```python
from build123d import *

# Parameters (mm, degrees)
PAD008_DEPTH      = 9.5
POCKET004_DEPTH   = 7
POCKET005_DEPTH   = 7.3
PAD009_DEPTH      = 4.1
PAD009_DEPTH_BACK = 9.5
PAD010_DEPTH      = 9.5
SKETCH019_R       = 2.1
PAD011_DEPTH      = 3


with BuildPart() as part:
    # Sketch012 → Pad008 (new body, symmetric)
    with BuildSketch(Plane.YZ):
        Polygon((-50.2140974459, 25.1635701276), (-41.6041734691, 21.1486966411), (-32.9942494922, 17.1338231546), (-30.6406576873, 16.391738509), (-21.2849840337, 14.7420808212), (-11.9293103801, 13.0924231333), (-9.4638496319, 12.9847787924), (0, 13.8127583485), (9.4638496319, 14.6407379046), (11.8731622478, 15.1748696522), (20.8002421453, 18.4240610138), (29.7273220427, 21.6732523754), (31.9162958532, 22.8127600157), (39.698240274, 28.261736161), (47.4801846947, 33.7107123064), (49.7744904401, 30.4341041292), (34.2106015986, 19.5361518385), (31.0954026161, 17.9144818923), (13.2412428211, 11.4160991691), (9.8124726029, 10.6559591122), (-9.1152266609, 9), (-12.6239030908, 9.1531921213), (-31.335250398, 12.4525074969), (-34.6847225392, 13.5085920064), (-51.9045704929, 21.5383389795), align=None)
    extrude(amount=PAD008_DEPTH, both=True)

    # Sketch013 → Pocket004 (cut, symmetric)
    with BuildSketch(Plane.YZ):
        Polygon((45.432304584, 32.2767712155), (39.698240274, 28.261736161), (33.9641759639, 24.2467011065), (34.7671886347, 23.0998922076), (33.7022888371, 22.3542413419), (35.1935840518, 20.2244435621), (41.9925460194, 24.9851279839), (48.791507987, 29.7458124056), (47.3002178304, 31.8756137271), (46.2353203941, 31.1299645148), align=None)
        Polygon((27.3780904908, 20.8182020171), (20.8002421453, 18.4240610138), (14.2223937998, 16.0299200105), (14.701229209, 14.7143529651), (13.4796275966, 14.2697263401), (14.3688739661, 11.826523341), (22.1683227186, 14.6652905307), (29.9677714711, 17.5040577203), (29.078530336, 19.9472626244), (27.8569308195, 19.5026367622), align=None)
        Polygon((-6.9733628866, 13.2026681492), (-6.8513426496, 11.8079957641), (-8.1463884643, 11.6946939366), (-7.9197930232, 9.1045868913), (0.348622971, 9.8279795561), (8.6170389652, 10.5513722209), (8.390436117, 13.1414786182), (7.0953826538, 13.0281761215), (6.9733628866, 14.4228485477), (0, 13.8127583485), align=None)
        Polygon((-21.2849840337, 14.7420808212), (-28.1786383048, 15.9576180648), (-28.4217503954, 14.5788880291), (-29.701997863, 14.8046301996), (-30.1534810944, 12.2441296837), (-21.9795767444, 10.8028498091), (-13.8056723944, 9.3615699345), (-13.3541906242, 11.922070708), (-14.6344528215, 12.1478154758), (-14.3913297626, 13.5265435775), align=None)
        Polygon((-41.6041734691, 21.1486966411), (-47.9483279783, 24.1070244733), (-48.5400033464, 22.838198142), (-49.7182011739, 23.3876008118), (-50.8170011484, 21.0311970654), (-43.294646516, 17.523465493), (-35.7722918836, 14.0157339205), (-34.6734914189, 16.3721374383), (-35.8516963311, 16.9215434118), (-35.2600189598, 18.1903688089), align=None)
    extrude(amount=POCKET004_DEPTH, both=True, mode=Mode.SUBTRACT)

    # Sketch014 → Pocket005 (cut, symmetric)
    with BuildSketch(Plane.YZ):
        Polygon((27.8569308195, 19.5026367622), (27.7885250582, 19.6905746558), (14.6328241506, 14.9022911145), (14.701229209, 14.7143529651), (13.4796275966, 14.2697263401), (13.7532418641, 13.5179715711), (29.3521429929, 19.1955072693), (29.078530336, 19.9472626244), align=None)
        Polygon((7.0779512585, 13.2274150395), (7.0953826538, 13.0281761215), (8.390436117, 13.1414786182), (8.4601600703, 12.3445228037), (-8.0766667901, 10.8977379227), (-8.1463884643, 11.6946939366), (-6.8513426496, 11.8079957641), (-6.8687741121, 12.0072346763), align=None)
        Polygon((34.6524725388, 23.2637220503), (46.1206038498, 31.2937940434), (46.2353203941, 31.1299645148), (47.3002178304, 31.8756137271), (47.7590763401, 31.2202902435), (34.1611489031, 21.6989189481), (33.7022888371, 22.3542413419), (34.7671886347, 23.0998922076), align=None)
        Polygon((-48.5400033464, 22.838198142), (-49.7182011739, 23.3876008118), (-50.0562934738, 22.6625535052), (-35.0115838696, 15.6470902021), (-34.6734914189, 16.3721374383), (-35.8516963311, 16.9215434118), (-35.7671709924, 17.1028041826), (-48.4554782937, 23.0194590466), align=None)
        Polygon((-28.3870200967, 14.7758494628), (-28.4217503954, 14.5788880291), (-29.701997863, 14.8046301996), (-29.8409157804, 14.0167838869), (-13.4931080919, 11.1342243163), (-13.3541906242, 11.922070708), (-14.6344528215, 12.1478154758), (-14.5997209559, 12.3447766332), align=None)
    extrude(amount=POCKET005_DEPTH, both=True, mode=Mode.SUBTRACT)

    # Sketch017 → Pad009 (join, two sides)
    with BuildSketch(Plane.YZ) as pad009_sk:
        Polygon((-13.6657921568, 3.2443456032), (-12.6239030908, 9.1531921213), (-11.9293103801, 13.0924231333), (-9.4638496319, 12.9847787924), (-9.1152266609, 9), (-8.5922922044, 3.0228318115), (-8.5922922044, 0), (-13.6657921568, 0), align=None)
        Polygon((15.2933636811, 0), (10.3354070594, 0), (10.3354070594, 4.6787909237), (9.8124726029, 10.6559591122), (9.4638496319, 14.6407379046), (11.8731622478, 15.1748696522), (13.2412428211, 11.4160991691), (15.2933636811, 5.7779434443), align=None)
    extrude(amount=PAD009_DEPTH)
    extrude(pad009_sk.sketch, amount=-PAD009_DEPTH_BACK)

    # Sketch018 → Pad010 (join)
    with BuildSketch(Plane.YZ):
        with BuildLine():
            Line((-37.2204321096, 8.0707452842), (-34.6847225392, 13.5085920064))
            Line((-34.6847225392, 13.5085920064), (-32.9942494922, 17.1338231546))
            Line((-32.9942494922, 17.1338231546), (-30.6406576873, 16.391738509))
            Line((-30.6406576873, 16.391738509), (-31.335250398, 12.4525074969))
            Line((-31.335250398, 12.4525074969), (-32.377139464, 6.5436609789))
            Line((-32.377139464, 6.5436609789), (-35, 0))
            Line((-35, 0), (-45, 0))
            Line((-45, 0), (-45, 3))
            add(Edge.make_bspline(
                [(-37.2204321096, 8.0707452842), (-39.0096732627, 4.233705249), (-40, 3), (-45, 3)],
                knots=[0, 0, 0, 0, 1, 1, 1, 1], degree=3))
        make_face()
        with BuildLine():
            Line((33.147523476, 12.2763261675), (31.0954026161, 17.9144818923))
            Line((31.0954026161, 17.9144818923), (29.7273220427, 21.6732523754))
            Line((29.7273220427, 21.6732523754), (31.9162958532, 22.8127600157))
            Line((31.9162958532, 22.8127600157), (34.2106015986, 19.5361518385))
            Line((34.2106015986, 19.5361518385), (37.6520602168, 14.6212395727))
            add(Edge.make_bspline(
                [(37.6520602168, 14.6212395727), (42.262119346, 8.0373928164), (40, 3), (45, 3)],
                knots=[0, 0, 0, 0, 1, 1, 1, 1], degree=3))
            Line((45, 3), (45, 0))
            Line((45, 0), (35, 0))
            Line((35, 0), (33.147523476, 12.2763261675))
        make_face()
    extrude(amount=-PAD010_DEPTH)

    # Sketch019 → Pad011 (join)
    with BuildSketch(Plane.XY):
        with BuildLine():
            Line((7.6224992299, 46.0948753465), (0, 40))
            Line((0, 40), (0, 45))
            Line((0, 45), (-9.5, 45))
            Line((-9.5, 45), (-9.5, 55))
            Line((-9.5, 55), (4.5, 55))
            ThreePointArc((7.6224992299, 46.0948753465), (9.218348401, 51.6544450327), (4.5, 55))
        make_face()
        with Locations((0, 50)):
            Circle(SKETCH019_R, mode=Mode.SUBTRACT)
        with BuildLine():
            Line((0, -45), (0, -40))
            Line((0, -40), (7.6224992299, -46.0948753465))
            ThreePointArc((4.5, -55), (9.218348401, -51.6544450327), (7.6224992299, -46.0948753465))
            Line((4.5, -55), (-9.5, -55))
            Line((-9.5, -55), (-9.5, -45))
            Line((-9.5, -45), (0, -45))
        make_face()
        with Locations((0, -50)):
            Circle(SKETCH019_R, mode=Mode.SUBTRACT)
    extrude(amount=PAD011_DEPTH)


with BuildPart() as part_1:
    # Body002 placement: moved
    add(part.part.moved(Location((50, 0, 5))))


solid = part_1.part
```
Work out the finished part from the listing and answer in its coordinate system (mm). A direction names the side the tool comes from. Coordinates: 2 decimals unless noted, no trailing zeros. Order: outer loops, then holes, each group sorted by start corner. A loop starts at its lowest first (then second) coordinate and runs counter-clockwise, first axis right, second up. Notation, with made-up numbers: (77.25, -36.75) - (94.25, -36.75) arc R33 cw to (94.25, -1.75) - close; hole circle Ø11 at (-6, 70.25). An arc over 180 degrees is marked (long way). Answer as a JSON object with one key per item and string values.
1. Find section A-A on y = 24. Determine the outline of the cut face in (x, z).
Output values:
{"outline": "(40.5, 20.33) - (43, 20.33) - (43, 22.25) - (42.7, 22.25) - (42.7, 23.31) - (43, 23.31) - (43, 24.59) - (40.5, 24.59) - close; (57, 20.33) - (59.5, 20.33) - (59.5, 24.59) - (57, 24.59) - (57, 23.31) - (57.3, 23.31) - (57.3, 22.25) - (57, 22.25) - close"}
2. A tool of negligible diameter and unlimited length cuts with its end or side. For faces 1 (the face through (58.58, 42.1, 30.06)), 2 (the face through (42.7, -42.4, 24.5)), 3 (the face through (47, -13.666, 7)), 4 (the face through (54.1, -11, 10)), from which of +Z, -Z, +X, -X, +Y, -Y can it reach the whole face along a straight path? Write none if from no direction.
Output values:
{"face 1": "+X, -X, +Y", "face 2": "none", "face 3": "-Z, +X, -X", "face 4": "-Z, +X"}
3. Find section D-D on y = -10.5. Determine the outline of the cut face in (x, z).
Output values:
{"outline": "(40.5, 5) - (54.1, 5) - (54.1, 14.06) - (59.5, 14.06) - (59.5, 18.03) - (40.5, 18.03) - close"}
4. Consider line 1 (X direction, y = -23, z = 18); line 2 (Y direction, x = 45, z = 12.5); line 3 (Y direction, x = 43.75, z = 15). Determine where each line is inside the solid, lowest interval first.
Output values:
{"line 1": "x = 40.5 to 42.7, 57.3 to 59.5", "line 2": "y = -37.49 to -32.21, -12.92 to -8.98, 10.09 to 14.67, 33.87 to 40.84", "line 3": "y = -36.32 to -31.77, -13.69 to -8, 9.87 to 13.76, 33.49 to 40.05"}
5. Each of these flat-tipped pins is pushed along its axis until it touches: P1, Ø4, axis at y = -35, z = 8.5, coming from the +X side; P2, Ø1, axis at x = 57, y = -3.5, coming from the +Z side; P3, Ø6, axis at x = 43.5, z = 23, coming from the -Y side; P4, Ø10, axis at y = 20.5, z = 33.5, coming from the +X side. Where does it stop, or does it pass through?
Output values:
{"P1": "stops at x = 50", "P2": "stops at z = 18.55", "P3": "stops at y = -50.66", "P4": "passes through"}
6. The mould has two halves that part along Z. Classify faces 5 (the face through (50.133, 30.806, 27.235)), 6 (the face through (59.246, 51.573, 6.479)), 7 (the face through (50.1, 47.6, 8)), 8 (the face through (56.84, 11.55, 16.04)): +Z half, -Z half, draft (parallel to the pull), parting line (faces both ways), or undercut.
Output values:
{"face 5": "+Z half", "face 6": "draft", "face 7": "undercut", "face 8": "-Z half"}
7. Find section B-B on y = -38.5. Count the separate pieces of the cut face and the enclosed holes in it, plus the area to 3 significant figures.
Output values:
{"separate pieces": "3", "enclosed holes": "0", "area": "75.0 mm²"}
8. Find section C-C on y = 6. Determine the outline of the cut face in (x, z).
Output values:
{"outline": "(40.5, 15.32) - (43, 15.32) - (43, 17.13) - (42.7, 17.13) - (42.7, 18.13) - (43, 18.13) - (43, 19.34) - (40.5, 19.34) - close; (57, 15.32) - (59.5, 15.32) - (59.5, 19.34) - (57, 19.34) - (57, 18.13) - (57.3, 18.13) - (57.3, 17.13) - (57, 17.13) - close"}
